```python
from build123d import *

# Parameters (mm, degrees)
SKETCH1_W           = 76.2
SKETCH1_H           = 35.56
SKETCH1_R           = 2.667
BOSS_EXTRUDE1_DEPTH = 3.175
SKETCH2_R           = 1.3462
CUT_EXTRUDE1_DEPTH  = 6.35


with BuildPart() as part:
    # Sketch1 → Boss-Extrude1 (new, symmetric)
    with BuildSketch(Plane(origin=(0, 0, 0), x_dir=(1, 0, 0), z_dir=(0, 1, 0))):
        Rectangle(SKETCH1_W, SKETCH1_H)
        with Locations(Location((-25.4, 6.35, 0), (0, 0, 270))):
            Circle(SKETCH1_R, mode=Mode.SUBTRACT)
        with Locations(Location((-12.7, 6.35, 0), (0, 0, 270))):
            Circle(SKETCH1_R, mode=Mode.SUBTRACT)
        with Locations(Location((0, 6.35, 0), (0, 0, 270))):
            Circle(SKETCH1_R, mode=Mode.SUBTRACT)
        with Locations(Location((12.7, 6.35, 0), (0, 0, 270))):
            Circle(SKETCH1_R, mode=Mode.SUBTRACT)
        with Locations(Location((25.4, 6.35, 0), (0, 0, 270))):
            Circle(SKETCH1_R, mode=Mode.SUBTRACT)
        with Locations(Location((-12.7, -6.35, 0), (0, 0, 270))):
            Circle(SKETCH1_R, mode=Mode.SUBTRACT)
        with Locations(Location((0, -6.35, 0), (0, 0, 270))):
            Circle(SKETCH1_R, mode=Mode.SUBTRACT)
        with Locations(Location((12.7, -6.35, 0), (0, 0, 270))):
            Circle(SKETCH1_R, mode=Mode.SUBTRACT)
        with Locations(Location((25.4, -6.35, 0), (0, 0, 270))):
            Circle(SKETCH1_R, mode=Mode.SUBTRACT)
        with Locations(Location((-25.4, -6.35, 0), (0, 0, 270))):
            Circle(SKETCH1_R, mode=Mode.SUBTRACT)
    extrude(amount=BOSS_EXTRUDE1_DEPTH, both=True)

    # Sketch2 → Cut-Extrude1 (cut)
    with BuildSketch(Plane.ZY.offset(38.1)):
        with Locations((-12.7, 0)):
            Circle(SKETCH2_R)
        with Locations((-6.35, 0)):
            Circle(SKETCH2_R)
        Circle(SKETCH2_R)
        with Locations((6.35, 0)):
            Circle(SKETCH2_R)
        with Locations((12.7, 0)):
            Circle(SKETCH2_R)
    extrude(amount=-CUT_EXTRUDE1_DEPTH, mode=Mode.SUBTRACT)


solid = part.part
```
Part model, mm, in its own coordinate system. A direction names the side the tool comes from. Round coordinates to 2 decimals unless told otherwise and drop trailing zeros. Loops run counter-clockwise (first coordinate to the right, second up) from the corner with the lowest first, then second, coordinate; pieces in that order, holes last. Notation, with made-up numbers: (-26, -36) -> (-11, -36) arc R23 cw to (-11, -10) -> close; hole circle Ø8 at (88.25, 84). An arc over 180 degrees is marked (long way). Use CSV: the item, a comma, the result in double quotes. Start each with the question number.
1) Cut at C-C, the plane z = -7. Write the cut outline in (x, y) (3 decimals).
2) Drop flat-ended pins along their axis: P1, Ø3, axis at x = -25.4, z = 6.35, coming from the -Y side; P2, Ø1.3, axis at y = 0, z = 0.5, coming from the -X side. Give the stop position or say it passes through.
3) Cut at B-B, the plane z = 12.7. Write the cut outline in (x, y) (3 decimals).
4) Which spindle directions (+Z, -Z, +X, -X, +Y, -Y) get a long thin tool onto all of the face, cutting with end or side? Do faces 1 (the flat face through (-31.75, 0, 13)), 2 (the cylindrical face through (-1.021, -0.044, 8.814)). Say none if no direction does.
5) Wall check: L1, parallel to Z at x = 15, y = 2.25; L2, parallel to X at y = 1.5, z = 6.35; L3, parallel to Z at x = 25.5, y = -0.75. Give the ranges that are in metal, low to high. Write a range as [from, to].
6) Pull direction Y, two halves, no side cores. Call faces 3 (the flat face through (-31.75, 0, 0)), 4 (the cylindrical face through (-15.304, -0.044, -6.928)): +Y half, -Y half, draft (parallel to the pull), parting line (faces both ways), or undercut.
7) Cut at D-D, the plane z = 6. Write the cut outline in (x, y) (3 decimals), plus the area to 3 significant figures.
8) Cut at A-A, the plane x = 0. Write the cut outline in (y, z) (3 decimals), plus the area to 3 significant figures.
Determined:
1,outline,"(-38.1, -3.175) -> (-27.987, -3.175) -> (-27.987, 3.175) -> (-38.1, 3.175) -> (-38.1, 1.179) -> (-31.75, 1.179) -> (-31.75, -1.179) -> (-38.1, -1.179) -> close; (-22.813, -3.175) -> (-15.287, -3.175) -> (-15.287, 3.175) -> (-22.813, 3.175) -> close; (-10.113, -3.175) -> (-2.587, -3.175) -> (-2.587, 3.175) -> (-10.113, 3.175) -> close; (2.587, -3.175) -> (10.113, -3.175) -> (10.113, 3.175) -> (2.587, 3.175) -> close; (15.287, -3.175) -> (22.813, -3.175) -> (22.813, 3.175) -> (15.287, 3.175) -> close; (27.987, -3.175) -> (38.1, -3.175) -> (38.1, 3.175) -> (27.987, 3.175) -> close"
2,P1,"passes through"
2,P2,"stops at x = -31.75"
3,outline,"(-38.1, -3.175) -> (38.1, -3.175) -> (38.1, 3.175) -> (-38.1, 3.175) -> (-38.1, 1.346) -> (-31.75, 1.346) -> (-31.75, -1.346) -> (-38.1, -1.346) -> close"
4,face 1,"-X"
4,face 2,"+Y, -Y"
5,L1,"z = [-17.78, -7.7], [-5, 5], [7.7, 17.78]"
5,L2,"x = [-38.1, -28.07], [-22.73, -15.37], [-10.03, -2.67], [2.67, 10.03], [15.37, 22.73], [28.07, 38.1]"
5,L3,"z = [-17.78, -9.02], [-3.68, 3.68], [9.02, 17.78]"
6,face 3,"undercut"
6,face 4,"draft"
7,outline,"(-38.1, -3.175) -> (-28.044, -3.175) -> (-28.044, 3.175) -> (-38.1, 3.175) -> (-38.1, 1.3) -> (-31.75, 1.3) -> (-31.75, -1.3) -> (-38.1, -1.3) -> close; (-22.756, -3.175) -> (-15.344, -3.175) -> (-15.344, 3.175) -> (-22.756, 3.175) -> close; (-10.056, -3.175) -> (-2.644, -3.175) -> (-2.644, 3.175) -> (-10.056, 3.175) -> close; (2.644, -3.175) -> (10.056, -3.175) -> (10.056, 3.175) -> (2.644, 3.175) -> close; (15.344, -3.175) -> (22.756, -3.175) -> (22.756, 3.175) -> (15.344, 3.175) -> close; (28.044, -3.175) -> (38.1, -3.175) -> (38.1, 3.175) -> (28.044, 3.175) -> close"
7,area,"299 mm2"
8,outline,"(-3.175, -17.78) -> (3.175, -17.78) -> (3.175, -9.017) -> (-3.175, -9.017) -> close; (-3.175, -3.683) -> (3.175, -3.683) -> (3.175, 3.683) -> (-3.175, 3.683) -> close; (-3.175, 9.017) -> (3.175, 9.017) -> (3.175, 17.78) -> (-3.175, 17.78) -> close"
8,area,"158 mm2"
